Verification items for this drawing (mm, ordinates from the low corner). A direction names the side the tool comes from. Coordinates: 2 decimals unless noted, no trailing zeros. Write each loop counter-clockwise with the first axis right and the second up, starting at its lowest first coordinate (ties: lowest second). Pieces come first, ordered by that corner, then holes. Notation, with made-up numbers: (20, -25.5) -> (61, -25.5) arc R27 ccw to (61, -7.5) -> close; hole circle Ø4 at (71.5, 11). An arc over 180 degrees is marked (long way). One line per item, written item: value. Start each with the question number.
1) Draft check along Z on the marked faces 3, 4 and 5. Enter one of: +Z half, -Z half, draft (parallel to the pull), parting line (faces both ways), or undercut.
2) Sectioned sample at C-C on x = 45. Enter the section's corners in (y, z).
3) Sectioned sample at B-B on z = 5. Enter the section's corners in (x, y).
4) Set-up check for the marked faces 1 and 2: record each of +Z, -Z, +X, -X, +Y, -Y from which the full face is reachable in a straight line by a thin tool's end or side.
5) Sectioned sample at D-D on x = 20. Enter the section's corners in (y, z).
6) Gauge pin test, flat ends, axial feed: P1, Ø3.5, axis at x = 15, z = 5, coming from the -Y side; P2, Ø2.5, axis at x = 35, z = 5, coming from the +Y side. Record the tip position at first contact, or that the pin passes through.
7) Scan lines: line 1 along Y through (x, z) = (43, 2.75); line 2 along Z through (x, y) = (15, 0.65). Record each from-to range of solid material in increasing order. Write a range as [from, to].
8) Sectioned sample at A-A on y = 2. Enter the section's corners in (x, z), plus the area to 3 significant figures.
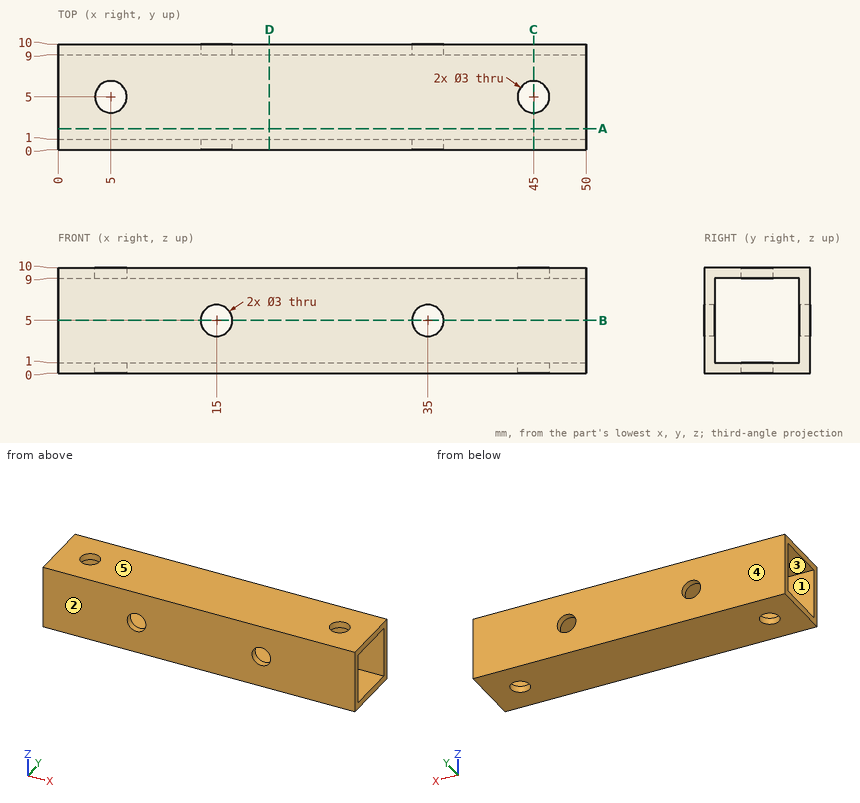
Answers:
1. face 3: undercut
1. face 4: draft
1. face 5: +Z half
2. outline: (0, 0) -> (3.5, 0) -> (3.5, 1) -> (1, 1) -> (1, 9) -> (3.5, 9) -> (3.5, 10) -> (0, 10) -> close; (6.5, 0) -> (10, 0) -> (10, 10) -> (6.5, 10) -> (6.5, 9) -> (9, 9) -> (9, 1) -> (6.5, 1) -> close
3. outline: (0, 0) -> (13.5, 0) -> (13.5, 1) -> (0, 1) -> close; (0, 9) -> (13.5, 9) -> (13.5, 10) -> (0, 10) -> close; (16.5, 0) -> (33.5, 0) -> (33.5, 1) -> (16.5, 1) -> close; (16.5, 9) -> (33.5, 9) -> (33.5, 10) -> (16.5, 10) -> close; (36.5, 0) -> (50, 0) -> (50, 1) -> (36.5, 1) -> close; (36.5, 9) -> (50, 9) -> (50, 10) -> (36.5, 10) -> close
4. face 1: +X, -X
4. face 2: +Z, -Z, +X, -X, -Y
5. outline: (0, 0) -> (10, 0) -> (10, 10) -> (0, 10) -> close; hole (1, 1) -> (9, 1) -> (9, 9) -> (1, 9) -> close
6. P1: stops at y = 0
6. P2: passes through
7. line 1: y = [0, 1], [9, 10]
7. line 2: z = [0, 3.5], [6.5, 10]
8. outline: (0, 0) -> (50, 0) -> (50, 1) -> (0, 1) -> close; (0, 9) -> (50, 9) -> (50, 10) -> (0, 10) -> close
8. area: 100 mm2
